from build123d import *

# Parameters (mm, degrees)
F0_W      = 76.2
F0_H      = 44.45
F1_DEPTH  = 25.4
F2_W      = 25.4
F2_H      = 31.75
F3_DEPTH  = 25.4
F4_R      = 6.35
F5_DEPTH  = 25.4
F6_R      = 6.35
F7_DEPTH  = 25.4
F9_DEPTH  = 25.4
F11_DEPTH = 25.4
F13_DEPTH = 25.4


with BuildPart() as f1:
    # F0 (on Front) → F1 (new body)
    with BuildSketch(Plane.XZ):
        with Locations((38.1, 22.225)):
            Rectangle(F0_W, F0_H)
    extrude(amount=F1_DEPTH)

    # F2 (on face) → F3 (cut)
    with BuildSketch(Plane.XZ.offset(25.4)):
        with Locations((12.7, 28.575)):
            Rectangle(F2_W, F2_H)
        with Locations((63.5, 28.575)):
            Rectangle(F2_W, F2_H)
    extrude(amount=-F3_DEPTH, mode=Mode.SUBTRACT)

    # F4 (on face) → F5 (cut)
    with BuildSketch(Plane.YZ.offset(50.8)):
        with Locations((-12.7, 31.75)):
            Circle(F4_R)
    extrude(amount=-F5_DEPTH, mode=Mode.SUBTRACT)

    # F6 (on face) → F7 (cut)
    with BuildSketch(Plane.XY.offset(12.7)):
        with Locations((12.7, -12.7)):
            Circle(F6_R)
        with Locations((63.5, -12.7)):
            Circle(F6_R)
    extrude(amount=-F7_DEPTH, mode=Mode.SUBTRACT)

    # F8 (on face) → F9 (cut)
    with BuildSketch(Plane.XY.offset(12.7)):
        with BuildLine():
            ThreePointArc((0, -12.7), (3.7197438789, -3.7197438789), (12.7, 0))
            Line((12.7, 0), (0, 0))
            Line((0, 0), (0, -12.7))
        make_face()
        with BuildLine():
            ThreePointArc((12.7, -25.4), (3.7197438789, -21.6802561211), (0, -12.7))
            Line((0, -12.7), (0, -25.4))
            Line((0, -25.4), (12.7, -25.4))
        make_face()
    extrude(amount=-F9_DEPTH, mode=Mode.SUBTRACT)

    # F10 (on face) → F11 (cut)
    with BuildSketch(Plane.XY.offset(12.7)):
        with BuildLine():
            ThreePointArc((63.5, 0), (75.7852064607, -12.7), (63.5, -25.4))
            Line((63.5, -25.4), (76.2, -25.4))
            Line((76.2, -25.4), (76.2, 0))
            Line((76.2, 0), (63.5, 0))
        make_face()
    extrude(amount=-F11_DEPTH, mode=Mode.SUBTRACT)

    # F12 (on face) → F13 (cut)
    with BuildSketch(Plane(origin=(25.4, 0, 0), x_dir=(0, -1, 0), z_dir=(-1, 0, 0))):
        with BuildLine():
            ThreePointArc((0, 31.7254364491), (12.5488484963, 44.2842424577), (25.4, 32.0349521935))
            Line((25.4, 32.0349521935), (25.4, 44.45))
            Line((25.4, 44.45), (0, 44.45))
            Line((0, 44.45), (0, 31.7254364491))
        make_face()
    extrude(amount=-F13_DEPTH, mode=Mode.SUBTRACT)


solid = f1.part
Could you check a few things on this model? Use its own coordinates, in mm. A direction names the side the tool comes from. Give positions to 0.01 mm unless a question says otherwise; leave off trailing zeros. Order: outer loops, then holes, each group sorted by start corner. A loop starts at its lowest first (then second) coordinate and runs counter-clockwise, first axis right, second up. Notation, with made-up numbers: (28, 77.25) -> (45, 77.25) arc R19 cw to (45, 94.25) -> close; hole circle Ø1 at (74, 22). An arc over 180 degrees is marked (long way). Answer in a Markdown table with one row per item. Add a question column.
Item 1: We'd pull the mould along Z, two halves only. Please class faces 3 (the cylindrical face through (38.278, -6.643, 33.657)), 4 (the flat face through (50.8, -13, 25)), 5 (the flat face through (57.6, -15.7, 12.7)): pulls with the +Z half, pulls with the -Z half, needs draft (parallel to the pull), parting line crosses it, or undercut.
Item 2: Imagine slicing it at B-B (x = 16). List the corners of the cut face in (y, z) for me, and give its area (3 significant figures).
Item 3: Imagine slicing it at D-D (z = 36). List the corners of the cut face in (x, y) for me.
Item 4: Imagine slicing it at C-C (y = -10.5). List the corners of the cut face in (x, z) for me.
Item 5: Imagine slicing it at A-A (z = 11.5). List the corners of the cut face in (x, y) for me.
Item 6: Please list where these lines run through material, in increasing order: probe 1 along X at (y, z) = (-7.75, 6.5); probe 2 along Z at (x, y) = (21, -16.5); probe 3 along Y at (x, z) = (35, 27).
Item 7: For faces 1 (the cylindrical face through (37.922, -12.274, 44.278)), 2 (the flat face through (15, -19, 12.7)), which set-ups out of +Z, -Z, +X, -X, +Y, -Y let a thin tool reach every point of the face, with its end or its side?
Item 8: I'm going to push flat-ended pins straight in: P1, Ø10, axis at x = 60.5, y = -10.5, coming from the -Z side; P2, Ø6, axis at y = -13.5, z = 39, coming from the -X side. Where does each tip first touch, or does it pass through?
Result:
| question | item | result |
|---|---|---|
| 1 | face 3 | undercut |
| 1 | face 4 | needs draft |
| 1 | face 5 | pulls with the +Z half |
| 2 | outline | (-25.4, 0) -> (-18.13, 0) -> (-18.13, 12.7) -> (-25.4, 12.7) -> close; (-7.27, 0) -> (0, 0) -> (0, 12.7) -> (-7.27, 12.7) -> close |
| 2 | area | 185 mm2 |
| 3 | outline | (25.4, -24.61) -> (50.8, -24.61) -> (50.8, -17.42) -> (25.4, -17.42) -> close; (25.4, -7.98) -> (50.8, -7.98) -> (50.8, -0.79) -> (25.4, -0.79) -> close |
| 4 | outline | (0.19, 0) -> (6.74, 0) -> (6.74, 12.7) -> (0.19, 12.7) -> close; (18.66, 0) -> (57.54, 0) -> (57.54, 12.7) -> (50.8, 12.7) -> (50.8, 25.79) -> (25.4, 25.79) -> (25.4, 12.7) -> (18.66, 12.7) -> close; (25.4, 37.71) -> (50.8, 37.71) -> (50.8, 44.09) -> (25.4, 44.09) -> close; (69.46, 0) -> (75.59, 0) -> (75.59, 12.7) -> (69.46, 12.7) -> close |
| 5 | outline | (12.7, -25.4) -> (63.5, -25.4) arc R12.71 ccw to (63.5, 0) -> (12.7, 0) arc R12.7 ccw to start; hole circle Ø12.7 at (12.7, -12.7); hole circle Ø12.7 at (63.5, -12.7) |
| 6 | probe 1 | 1 to 8.72, 16.68 to 59.52, 67.48 to 74.78 |
| 6 | probe 2 | 0 to 12.7 |
| 6 | probe 3 | -25.4 to -16.91, -8.49 to 0 |
| 7 | face 1 | +Z, +X, -X |
| 7 | face 2 | +Z, -X, +Y, -Y |
| 8 | P1 | z = 0 |
| 8 | P2 | x = 25.4 |
